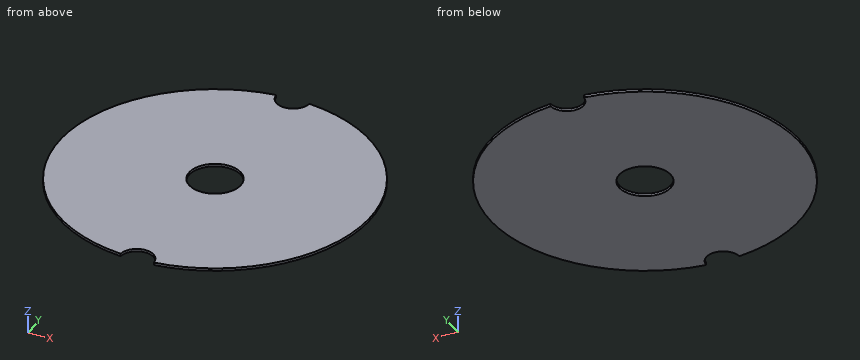
Autodesk Inventor part; units mm, degrees
ref_plane "YZ Plane" through (0, 0, 0) normal (1, 0, 0) x (0, 1, 0)
ref_plane "XZ Plane" through (0, 0, 0) normal (0, 1, 0) x (-1, 0, 0)
ref_plane "XY Plane" through (0, 0, 0) normal (0, 0, 1) x (1, 0, 0)
sketch "草圖1" plane through (0, 0, 0) normal (0, 0, 1) x (1, 0, 0)
  circle A0 centre (0, 0) radius 10
  dimension "d0" = 20
extrude "擠出1" add sketch "草圖1" along normal blind 17
sketch "草圖2" plane through (0, 0, 0) normal (0, 0, -1) x (-1, 0, 0)
  circle A0 centre (0, 0) radius 10
  circle A1 centre (0, 0) radius 60
  line L0 (0, 0) -> (0, 60)
  circle A2 centre (0, 60) radius 6.5
  dimension "d3" = 120
  dimension "d4" = 13
extrude "擠出2" add sketch "草圖2" along normal blind 1 contours A0 | A2 A1 | A2 A1 L0 | L0 A1 A2 picked at (-11.4207, 38.8636)
extrude "擠出3" cut sketch "草圖2" along normal blind 1 contours A2 A1 L0 | L0 A1 A2 | A1 A2 picked at (1.4483, 62.0284)
pattern_circular "環形陣列1" count 2 over 360 about axis through (0, 0, 0) along (0, 0, -1) of "擠出3"
sketch "草圖3" plane through (0, 0, 17) normal (0, 0, 1) x (1, 0, 0)
  circle A0 centre (0, 0) radius 10
extrude "擠出4" cut sketch "草圖3" against normal blind 65
Here's how the part is built. I have some questions about the finished solid (model axes, mm). Round coordinates to 2 decimals unless told otherwise and drop trailing zeros. Loops run counter-clockwise (first coordinate to the right, second up) from the corner with the lowest first, then second, coordinate; pieces in that order, holes last. Notation, with made-up numbers: M -1.5,-5 L 25.5,-5 A25 ccw 25.5,32 Z; hole C -26,39 d5. An arc over 180 degrees is marked long. Write each question's results on one line, items separated by ' | '. Start each with the question number.
(1) If I drill on probe 1 along X at (y, z) = (7, -0.8); probe 2 along X at (y, z) = (-8, -0.5); probe 3 along X at (y, z) = (19, -0.4), over which ranges is the centre line in solid material (lowest first)? Write a range as from..to.
(2) Will this pin go through, and if not, where does the flat tip stop? P1, Ø12, axis at x = -17.5, y = 3.5, coming from the +Z side.
(3) I want a section at C-C (z = -0.55). Please give me the cut outline in (x, y).
(4) I want a section at A-A (y = 0). Please give me the cut outline in (x, z).
(5) I want a section at B-B (x = 0). Please give me the cut outline in (y, z).
(6) I want a section at D-D (y = 46.5). Please give me the cut outline in (x, z).
Solved:
1) probe 1: x = -59.59..-7.14, 7.14..59.59 | probe 2: x = -59.46..-6, 6..59.46 | probe 3: x = -56.91..56.91
2) P1: stops at z = 0
3) outline: M -6.49,-59.65 A6.5 cw 6.49,-59.65 A60 ccw 6.49,59.65 A6.5 cw -6.49,59.65 A60 ccw Z; hole C 0,0 d20
4) outline: M -60,-1 L -10,-1 L -10,0 L -60,0 Z; M 10,-1 L 60,-1 L 60,0 L 10,0 Z
5) outline: M -53.5,-1 L -10,-1 L -10,0 L -53.5,0 Z; M 10,-1 L 53.5,-1 L 53.5,0 L 10,0 Z
6) outline: M -37.92,-1 L 37.92,-1 L 37.92,0 L -37.92,0 Z
